Here's how the part is built. I have some questions about the finished solid (model axes, mm). Face numbers are marked on the shaded views. A direction names the side the tool comes from. Give positions to 0.01 mm unless a question says otherwise; leave off trailing zeros. Loops run counter-clockwise (first coordinate to the right, second up) from the corner with the lowest first, then second, coordinate; pieces in that order, holes last.
Q1. Suppose I cut it at D-D (x = 191.5). List the corners of the cut face in (y, z) for me.
Q2. Suppose I cut it at C-C (x = 117). List the corners of the cut face in (y, z) for me, and give its area (3 significant figures).
Q3. For the marked faces 5 and 6, which set-ups out of +Z, -Z, +X, -X, +Y, -Y let a thin tool reach every point of the face, with its end or its side?
Q4. Thinking about a two-plate mould opening in Z: for the marked faces 1, 2, 3 and 4, which applies, pulls with the +Z half, pulls with the -Z half, needs draft (parallel to the pull), parting line crosses it, or undercut?
Q5. I'm going to push flat-ended pins straight in: P1, Ø2, axis at x = 153, z = 38, coming from the +Y side; P2, Ø6, axis at y = 16, z = 99, coming from the -X side; P3, Ø17, axis at y = 56.5, z = 97.86, coming from the +X side; P4, Ø10, axis at y = 16.5, z = -41.5, coming from the +X side. Where does each tip first touch, or does it pass through?
Q6. I need wall thicknesses on probe 1 along Y at (x, z) = (266.5, 0); probe 2 along Z at (x, y) = (259, 56); probe 3 along X at (y, z) = (86.5, 70). Which ranges of each line are inside material? Lowest first, please.
Q7. Suppose I cut it at A-A (z = 113). List the corners of the cut face in (x, y) for me.
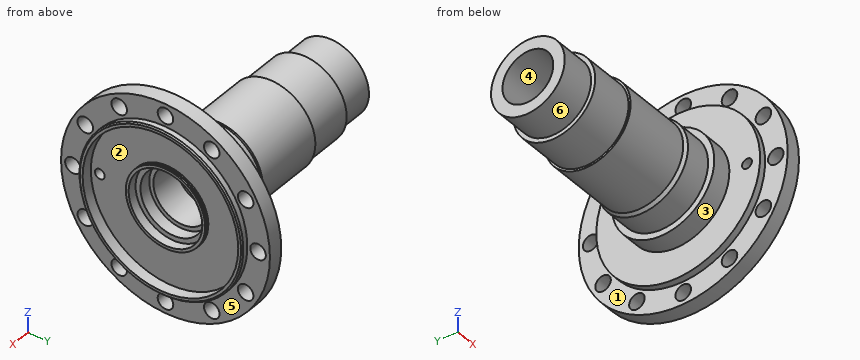
```python
from build123d import *

# Parameters (mm, degrees)
SKETCH_3_W           = 2
SKETCH_3_H           = 46.5
SKETCH_5_W           = 2
SKETCH_5_H           = 46.5
SKETCH_6_R           = 9.5
CUT_EXTRUDE_1_DEPTH  = 328.171973127
SKETCH_7_R           = 9.5
CUT_EXTRUDE_2_DEPTH  = 328.171973127
SKETCH_8_R           = 9.5
CUT_EXTRUDE_3_DEPTH  = 328.171973127
SKETCH_9_R           = 9.5
CUT_EXTRUDE_4_DEPTH  = 328.171973127
SKETCH_10_R          = 9.5
CUT_EXTRUDE_5_DEPTH  = 328.171973127
SKETCH_11_R          = 9.5
CUT_EXTRUDE_6_DEPTH  = 328.171973127
SKETCH_12_R          = 9.5
CUT_EXTRUDE_7_DEPTH  = 328.171973127
SKETCH_13_R          = 9.5
CUT_EXTRUDE_8_DEPTH  = 328.171973127
SKETCH_14_R          = 9.5
CUT_EXTRUDE_9_DEPTH  = 328.171973127
SKETCH_15_R          = 9.5
CUT_EXTRUDE_10_DEPTH = 328.171973127
SKETCH_16_R          = 9.5
CUT_EXTRUDE_11_DEPTH = 328.171973127
SKETCH_17_R          = 9.5
CUT_EXTRUDE_12_DEPTH = 328.171973127
SKETCH_18_R          = 6
CUT_EXTRUDE_13_DEPTH = 328.171973127


with BuildPart() as part:
    # Эскиз1 → Повернуть1 (revolve)
    with BuildSketch(Plane.XY, mode=Mode.PRIVATE) as revolve_1_sk:
        Polygon((0, 0), (273, 0), (273, 98.4), (271.4, 100), (265, 100), (265, 127.5), (247, 127.5), (247, 100), (239, 100), (239, 62.5), (215, 62.5), (215, 55), (183, 55), (178.669872981, 52.5), (95, 52.5), (95, 50), (42, 50), (42, 45), (0, 45), align=None)
    revolve(revolve_1_sk.sketch.rotate(Axis((0, 0, 0), (1, 0, 0)), 90), axis=Axis((0, 0, 0), (1, 0, 0)))

    # Эскиз2 → Вырез-Повернуть1 (revolve, cut)
    with BuildSketch(Plane.XY, mode=Mode.PRIVATE) as cut_revolve_1_sk:
        Polygon((0, 0), (273, 0), (273, 95), (265, 95), (265, 45), (254, 45), (254, 39), (240, 39), (240, 34), (203.5, 34), (203.5, 31), (0, 31), align=None)
    revolve(cut_revolve_1_sk.sketch.rotate(Axis((0, 0, 0), (1, 0, 0)), 90), axis=Axis((0, 0, 0), (1, 0, 0)), mode=Mode.SUBTRACT)

    # Эскиз3 → Rear_recess_left (revolve, cut)
    with BuildSketch(Plane.XY, mode=Mode.PRIVATE) as rear_recess_left_sk:
        with Locations((261, 71.75)):
            Rectangle(SKETCH_3_W, SKETCH_3_H)
    revolve(rear_recess_left_sk.sketch.rotate(Axis((0, 0, 0), (1, 0, 0)), 90), axis=Axis((0, 0, 0), (1, 0, 0)), mode=Mode.SUBTRACT)

    # Эскиз4 → Collar_groove_nominal (revolve, cut)
    with BuildSketch(Plane.XY, mode=Mode.PRIVATE) as collar_groove_nominal_sk:
        with BuildLine():
            Line((263, 48), (263, 95))
            Line((263, 95), (262, 95))
            Line((262, 95), (262, 48))
            ThreePointArc((262, 48), (262.146446609, 47.646446609), (262.5, 47.5))
            ThreePointArc((262.5, 47.5), (262.853553391, 47.646446609), (263, 48))
        make_face()
    revolve(collar_groove_nominal_sk.sketch.rotate(Axis((0, 0, 0), (1, 0, 0)), 90), axis=Axis((0, 0, 0), (1, 0, 0)), mode=Mode.SUBTRACT)

    # Эскиз5 → Rear_recess_lip (revolve, cut)
    with BuildSketch(Plane.XY, mode=Mode.PRIVATE) as rear_recess_lip_sk:
        with Locations((264, 71.75)):
            Rectangle(SKETCH_5_W, SKETCH_5_H)
    revolve(rear_recess_lip_sk.sketch.rotate(Axis((0, 0, 0), (1, 0, 0)), 90), axis=Axis((0, 0, 0), (1, 0, 0)), mode=Mode.SUBTRACT)

    # Эскиз6 → Вырез-Вытянуть1 (cut, through all)
    with BuildSketch(Plane(origin=(0, 0, 0), x_dir=(0, 0, -1), z_dir=(1, 0, 0))):
        with Locations(Location((0, 113, 0), (0, 0, 180))):
            Circle(SKETCH_6_R)
    extrude(amount=CUT_EXTRUDE_1_DEPTH, mode=Mode.SUBTRACT)

    # Эскиз7 → Вырез-Вытянуть2 (cut, through all)
    with BuildSketch(Plane(origin=(0, 0, 0), x_dir=(0, 0, -1), z_dir=(1, 0, 0))):
        with Locations(Location((-56.5, 97.860870628, 0), (0, 0, 180))):
            Circle(SKETCH_7_R)
    extrude(amount=CUT_EXTRUDE_2_DEPTH, mode=Mode.SUBTRACT)

    # Эскиз8 → Вырез-Вытянуть3 (cut, through all)
    with BuildSketch(Plane(origin=(0, 0, 0), x_dir=(0, 0, -1), z_dir=(1, 0, 0))):
        with Locations(Location((-97.860870628, 56.5, 0), (0, 0, 180))):
            Circle(SKETCH_8_R)
    extrude(amount=CUT_EXTRUDE_3_DEPTH, mode=Mode.SUBTRACT)

    # Эскиз9 → Вырез-Вытянуть4 (cut, through all)
    with BuildSketch(Plane(origin=(0, 0, 0), x_dir=(0, 0, -1), z_dir=(1, 0, 0))):
        with Locations(Location((-113, 0, 0), (0, 0, 180))):
            Circle(SKETCH_9_R)
    extrude(amount=CUT_EXTRUDE_4_DEPTH, mode=Mode.SUBTRACT)

    # Эскиз10 → Вырез-Вытянуть5 (cut, through all)
    with BuildSketch(Plane(origin=(0, 0, 0), x_dir=(0, 0, -1), z_dir=(1, 0, 0))):
        with Locations(Location((-97.860870628, -56.5, 0), (0, 0, 180))):
            Circle(SKETCH_10_R)
    extrude(amount=CUT_EXTRUDE_5_DEPTH, mode=Mode.SUBTRACT)

    # Эскиз11 → Вырез-Вытянуть6 (cut, through all)
    with BuildSketch(Plane(origin=(0, 0, 0), x_dir=(0, 0, -1), z_dir=(1, 0, 0))):
        with Locations(Location((-56.5, -97.860870628, 0), (0, 0, 180))):
            Circle(SKETCH_11_R)
    extrude(amount=CUT_EXTRUDE_6_DEPTH, mode=Mode.SUBTRACT)

    # Эскиз12 → Вырез-Вытянуть7 (cut, through all)
    with BuildSketch(Plane(origin=(0, 0, 0), x_dir=(0, 0, -1), z_dir=(1, 0, 0))):
        with Locations(Location((0, -113, 0), (0, 0, 180))):
            Circle(SKETCH_12_R)
    extrude(amount=CUT_EXTRUDE_7_DEPTH, mode=Mode.SUBTRACT)

    # Эскиз13 → Вырез-Вытянуть8 (cut, through all)
    with BuildSketch(Plane(origin=(0, 0, 0), x_dir=(0, 0, -1), z_dir=(1, 0, 0))):
        with Locations(Location((56.5, -97.860870628, 0), (0, 0, 180))):
            Circle(SKETCH_13_R)
    extrude(amount=CUT_EXTRUDE_8_DEPTH, mode=Mode.SUBTRACT)

    # Эскиз14 → Вырез-Вытянуть9 (cut, through all)
    with BuildSketch(Plane(origin=(0, 0, 0), x_dir=(0, 0, -1), z_dir=(1, 0, 0))):
        with Locations(Location((97.860870628, -56.5, 0), (0, 0, 180))):
            Circle(SKETCH_14_R)
    extrude(amount=CUT_EXTRUDE_9_DEPTH, mode=Mode.SUBTRACT)

    # Эскиз15 → Вырез-Вытянуть10 (cut, through all)
    with BuildSketch(Plane(origin=(0, 0, 0), x_dir=(0, 0, -1), z_dir=(1, 0, 0))):
        with Locations(Location((113, 0, 0), (0, 0, 180))):
            Circle(SKETCH_15_R)
    extrude(amount=CUT_EXTRUDE_10_DEPTH, mode=Mode.SUBTRACT)

    # Эскиз16 → Вырез-Вытянуть11 (cut, through all)
    with BuildSketch(Plane(origin=(0, 0, 0), x_dir=(0, 0, -1), z_dir=(1, 0, 0))):
        with Locations(Location((97.860870628, 56.5, 0), (0, 0, 180))):
            Circle(SKETCH_16_R)
    extrude(amount=CUT_EXTRUDE_11_DEPTH, mode=Mode.SUBTRACT)

    # Эскиз17 → Вырез-Вытянуть12 (cut, through all)
    with BuildSketch(Plane(origin=(0, 0, 0), x_dir=(0, 0, -1), z_dir=(1, 0, 0))):
        with Locations(Location((56.5, 97.860870628, 0), (0, 0, 180))):
            Circle(SKETCH_17_R)
    extrude(amount=CUT_EXTRUDE_12_DEPTH, mode=Mode.SUBTRACT)

    # Эскиз18 → Вырез-Вытянуть13 (cut, through all)
    with BuildSketch(Plane(origin=(0, 0, 0), x_dir=(0, 0, -1), z_dir=(1, 0, 0))):
        with Locations((0, -84)):
            Circle(SKETCH_18_R)
    extrude(amount=CUT_EXTRUDE_13_DEPTH, mode=Mode.SUBTRACT)


solid = part.part
```
Solutions:
1. outline: circle Ø110 at (0, 0); hole circle Ø62 at (0, 0)
2. outline: circle Ø105 at (0, 0); hole circle Ø62 at (0, 0)
2. area: 5,640 mm2
3. face 5: +X
3. face 6: -X
4. face 1: needs draft
4. face 2: undercut
4. face 3: parting line crosses it
4. face 4: undercut
5. P1: stops at y = 37.25
5. P2: stops at x = 239
5. P3: passes through
5. P4: stops at x = 265
6. probe 1: y = -100 to -95, 95 to 100
6. probe 2: z = -114.54 to -107.35, -88.37 to 88.37, 107.35 to 114.54
6. probe 3: x = 247 to 265
7. outline: (247, -59.05) - (265, -59.05) - (265, -9.5) - (247, -9.5) - close; (247, 9.5) - (265, 9.5) - (265, 59.05) - (247, 59.05) - close
